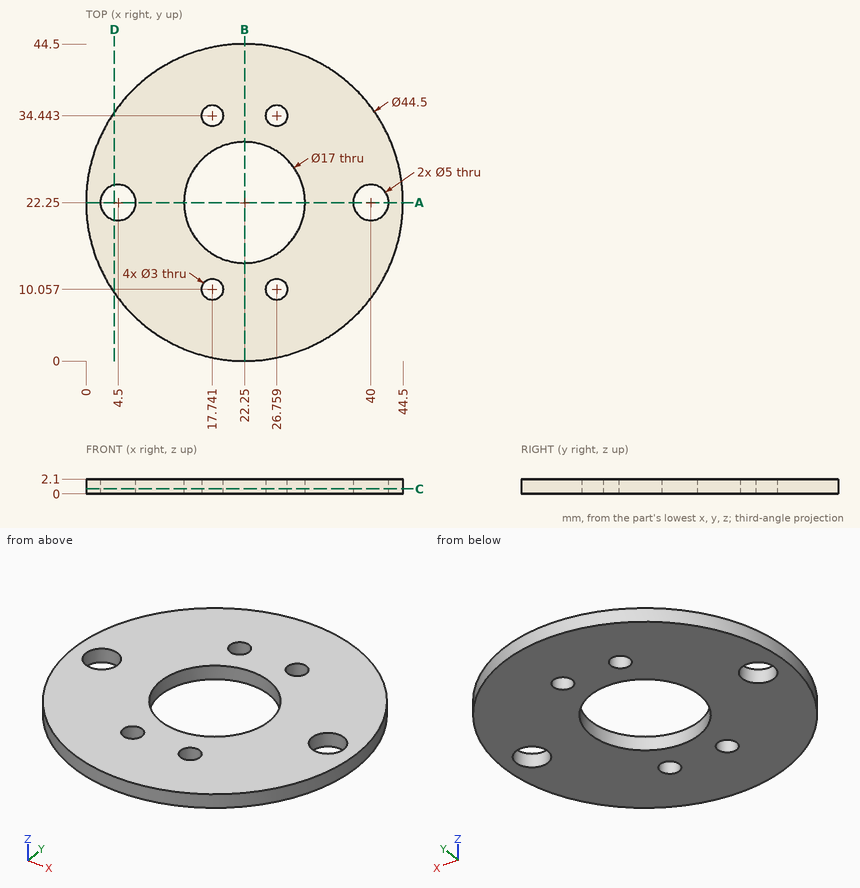
Could you check a few things on this drawing? It's one solid part, dimensions in mm from its lowest x, y, z. Round coordinates to 2 decimals unless told otherwise and drop trailing zeros. Order: outer loops, then holes, each group sorted by start corner. A loop starts at its lowest first (then second) coordinate and runs counter-clockwise, first axis right, second up. Notation, with made-up numbers: M -20.75,-15.5 L 36.25,-15.5 A23 ccw 36.25,15.5 Z; hole C -19,-15 d11. An arc over 180 degrees is marked long. Return JSON: item names as keys, results as strings. Group by question number.
1. If we section it at A-A on y = 22.25: List the corners of the cut face in (x, z) for me.
2. Please list where these lines run through material, in increasing order: probe 1 along X at (y, z) = (34, 1.2) (1 decimal); probe 2 along X at (y, z) = (34.5, 2) (1 decimal); probe 3 along Y at (x, z) = (19, 0.3) (1 decimal).
3. If we section it at B-B on x = 22.25: List the corners of the cut face in (y, z) for me.
4. If we section it at D-D on x = 4: List the corners of the cut face in (y, z) for me.
5. I'm going to push flat-ended pins straight in: pin 1 Ø4.5 at (x, y) = (4.5, 22.25) entering from +Z; pin 2 Ø1 at (y, z) = (10.5, 0.5) entering from -X; pin 3 Ø1 at (x, z) = (11.5, 1.5) entering from -Y. Where does each tip first touch, or does it pass through?
6. If we section it at C-C on z = 0.7: List the corners of the cut face in (x, y) for me.
Reply:
{
 "1": {"outline": "M 0,0 L 2,0 L 2,2.1 L 0,2.1 Z; M 7,0 L 13.75,0 L 13.75,2.1 L 7,2.1 Z; M 30.75,0 L 37.5,0 L 37.5,2.1 L 30.75,2.1 Z; M 42.5,0 L 44.5,0 L 44.5,2.1 L 42.5,2.1 Z"},
 "2": {"probe 1": "3.4 to 16.3, 19.2 to 25.3, 28.2 to 41.1", "probe 2": "3.7 to 16.2, 19.2 to 25.3, 28.3 to 40.8", "probe 3": "0.2 to 9.2, 10.9 to 14.4, 30.1 to 33.6, 35.3 to 44.3"},
 "3": {"outline": "M 0,0 L 13.75,0 L 13.75,2.1 L 0,2.1 Z; M 30.75,0 L 44.5,0 L 44.5,2.1 L 30.75,2.1 Z"},
 "4": {"outline": "M 9.52,0 L 19.8,0 L 19.8,2.1 L 9.52,2.1 Z; M 24.7,0 L 34.98,0 L 34.98,2.1 L 24.7,2.1 Z"},
 "5": {"pin 1": "through", "pin 2": "x = 3.05", "pin 3": "y = 2.5"},
 "6": {"outline": "C 22.25,22.25 d44.5; hole C 4.5,22.25 d5; hole C 22.25,22.25 d17; hole C 17.74,10.06 d3; hole C 17.74,34.44 d3; hole C 26.76,10.06 d3; hole C 26.76,34.44 d3; hole C 40,22.25 d5"}
}
